Source: CAD feature listing. Evaluate the final solid. Frame: model axes, mm. A direction names the side the tool comes from. Give positions to 0.01 mm unless a question says otherwise; leave off trailing zeros. Loops run counter-clockwise (first coordinate to the right, second up) from the corner with the lowest first, then second, coordinate; pieces in that order, holes last. Notation, with made-up numbers: M 38,79 L 45,79 A30 ccw 45,112 Z; hole C 12.5,2 d2. An arc over 180 degrees is marked long. Write item = value, one per line.
from build123d import *

# Parameters (mm, degrees)
BOSS_EXTRUDE1_DEPTH = 12.5
CUT_EXTRUDE1_REACH  = 50.719
SKETCH3_R           = 3
CUT_EXTRUDE2_DEPTH  = 3
SKETCH4_R           = 5.5
CUT_EXTRUDE3_DEPTH  = 5
FILLET1_R           = 5
SKETCH5_R           = 1.75
CUT_EXTRUDE4_DEPTH  = 9.1


with BuildPart() as part:
    # Sketch1 → Boss-Extrude1 (new body)
    with BuildSketch(Plane.XY):
        Polygon((-3.5, 31.5), (-17.5, 17.5), (-17.5, -17.5), (-3.5, -31.5), (3.5, -31.5), (17.5, -17.5), (17.5, 17.5), (3.5, 31.5), align=None)
    extrude(amount=BOSS_EXTRUDE1_DEPTH)

    # Sketch2 → Cut-Extrude1 (cut, up to next)
    with BuildSketch(Plane(origin=(17.5, 0, 0), x_dir=(0, 0, -1), z_dir=(1, 0, 0)), mode=Mode.PRIVATE) as cut_extrude1_sk1:
        with BuildLine():
            Line((-12.5, -7.495832175), (-12.5, 7.495832175))
            ThreePointArc((-12.5, 7.495832175), (-5.25, 0), (-12.5, -7.495832175))
        make_face()
    cut_extrude1_tool1 = extrude(cut_extrude1_sk1.sketch, amount=-CUT_EXTRUDE1_REACH, mode=Mode.PRIVATE) & part.part
    add(cut_extrude1_tool1.solids().sort_by_distance((17.5, 0, 9.431384))[0], mode=Mode.SUBTRACT)

    # Sketch3 → Cut-Extrude2 (cut)
    with BuildSketch(Plane(origin=(0, 0, 0), x_dir=(-1, 0, 0), z_dir=(0, 0, -1))):
        with Locations((-12.5, 12.5)):
            Circle(SKETCH3_R)
        with Locations(Location((12.5, 12.5, 0), (0, 0, 180))):
            Circle(SKETCH3_R)
        with Locations((12.5, -12.5)):
            Circle(SKETCH3_R)
        with Locations(Location((-12.5, -12.5, 0), (0, 0, 180))):
            Circle(SKETCH3_R)
    extrude(amount=-CUT_EXTRUDE2_DEPTH, mode=Mode.SUBTRACT)

    # Sketch4 → Cut-Extrude3 (cut)
    with BuildSketch(Plane.XY.offset(12.5)):
        with Locations((0, 22.5)):
            Circle(SKETCH4_R)
        with Locations(Location((0, -22.5, 0), (0, 0, 180))):
            Circle(SKETCH4_R)
    extrude(amount=-CUT_EXTRUDE3_DEPTH, mode=Mode.SUBTRACT)

    # Fillet1
    fillet1_edges = [part.edges().sort_by_distance(p)[0] for p in [
        (3.5, 31.5, 6.25),
        (17.5, 17.5, 6.25),
        (17.5, -17.5, 6.25),
        (3.5, -31.5, 6.25),
        (-3.5, -31.5, 6.25),
        (-17.5, -17.5, 6.25),
        (-17.5, 17.5, 6.25),
        (-3.5, 31.5, 6.25),
    ]]
    fillet(fillet1_edges, radius=FILLET1_R)

    # Sketch5 → Cut-Extrude4 (cut)
    with BuildSketch(Plane.XY.offset(12.5)):
        with Locations((-12.5, 12.5)):
            Circle(SKETCH5_R)
        with Locations(Location((12.5, 12.5, 0), (0, 0, 180))):
            Circle(SKETCH5_R)
        with Locations((12.5, -12.5)):
            Circle(SKETCH5_R)
        with Locations(Location((-12.5, -12.5, 0), (0, 0, 180))):
            Circle(SKETCH5_R)
    extrude(amount=-CUT_EXTRUDE4_DEPTH, mode=Mode.SUBTRACT)


solid = part.part
1. Reachability of faces 1 (the flat face through (-13, 13, 3.4)), 2 (the flat face through (-11, -24, 6)), 3 (the flat face through (13, 13, 3)) from +Z, -Z, +X, -X, +Y, -Y: full face, straight path, thin tool, end or side. Return the list, or none.
Derived:
face_1 = +Z
face_2 = +Z, -Z, -X, -Y
face_3 = -Z
2. Cut plane A-A, the plane z = 2.25. Return the cut outline in (x, y).
Derived:
outline = M -17.5,-15.43 A5 ccw -16.04,-18.96 L -4.96,-30.04 A5 ccw -1.43,-31.5 L 1.43,-31.5 A5 ccw 4.96,-30.04 L 16.04,-18.96 A5 ccw 17.5,-15.43 L 17.5,15.43 A5 ccw 16.04,18.96 L 4.96,30.04 A5 ccw 1.43,31.5 L -1.43,31.5 A5 ccw -4.96,30.04 L -16.04,18.96 A5 ccw -17.5,15.43 Z; hole C -12.5,-12.5 d6; hole C -12.5,12.5 d6; hole C 12.5,-12.5 d6; hole C 12.5,12.5 d6
3. Material intervals for probe 1 along Y at (x, z) = (-14, 11); probe 2 along Y at (x, z) = (-13.5, 6.5); probe 3 along Z at (x, y) = (2, 22.5), sorted ascending. Write a range as from..to.
Derived:
probe_1 = -21..-13.4, -11.6..-7.29, 7.29..11.6, 13.4..21
probe_2 = -21.5..-13.94, -11.06..-4.15, 4.15..11.06, 13.94..21.5
probe_3 = 0..7.5
4. Pull-direction query (Y, two-part tool) for faces 4 (the cylindrical face through (17.13, -17.32, 6.34)), 5 (the cylindrical face through (-10.1, -14.3, 1.5)), 6 (the cylindrical face through (-3.37, 31.11, 6.34)); classes: +Y half, -Y half, draft (parallel to the pull), parting line (faces both ways), or undercut.
Derived:
face_4 = -Y half
face_5 = undercut
face_6 = +Y half
5. Cut plane D-D, the plane z = 10.5. Return the cut outline in (x, y).
Derived:
outline = M -17.5,-15.43 A5 ccw -16.04,-18.96 L -4.96,-30.04 A5 ccw -1.43,-31.5 L 1.43,-31.5 A5 ccw 4.96,-30.04 L 16.04,-18.96 A5 ccw 17.5,-15.43 L 17.5,-7.15 L -17.5,-7.15 Z; M -17.5,7.15 L 17.5,7.15 L 17.5,15.43 A5 ccw 16.04,18.96 L 4.96,30.04 A5 ccw 1.43,31.5 L -1.43,31.5 A5 ccw -4.96,30.04 L -16.04,18.96 A5 ccw -17.5,15.43 Z; hole C -12.5,-12.5 d3.5; hole C -12.5,12.5 d3.5; hole C 0,-22.5 d11; hole C 0,22.5 d11; hole C 12.5,-12.5 d3.5; hole C 12.5,12.5 d3.5
6. First-contact query: pin 1 Ø2 at (x, y) = (-12.5, -12.5) entering from +Z; pin 2 Ø3 at (x, z) = (3.5, 8) entering from +Y; pin 3 Ø5.5 at (x, y) = (-12.5, -12.5) entering from -Z. Flat tips, straight axial feed; report the tip coordinate or a pass-through.
Derived:
pin_1 = 3.4
pin_2 = 31.47
pin_3 = 3
7. Cut plane C-C, the plane y = -12.5. Return the cut outline in (x, z), then the cut area to 3 significant figures.
Derived:
outline = M -17.5,0 L -15.5,0 L -15.5,3 L -9.5,3 L -9.5,0 L 9.5,0 L 9.5,3 L 15.5,3 L 15.5,0 L 17.5,0 L 17.5,12.5 L 14.25,12.5 L 14.25,3.4 L 10.75,3.4 L 10.75,12.5 L -10.75,12.5 L -10.75,3.4 L -14.25,3.4 L -14.25,12.5 L -17.5,12.5 Z
area = 338 mm²
